Here's how the part is built. I have some questions about the finished solid (model axes, mm). A direction names the side the tool comes from. Give positions to 0.01 mm unless a question says otherwise; leave off trailing zeros. Order: outer loops, then holes, each group sorted by start corner. A loop starts at its lowest first (then second) coordinate and runs counter-clockwise, first axis right, second up.
from build123d import *

# Parameters (mm, degrees)
SKETCH1_R               = 8.2
BOSS_EXTRUDE1_DEPTH     = 72
SKETCH2_R               = 2.6
CUT_EXTRUDE1_DEPTH      = 6
CHAMFER1_SIZE           = 0.5
CHAMFER2_SIZE           = 1
SKETCH3_R               = 2.6
CUT_EXTRUDE2_DEPTH      = 33
CUT_EXTRUDE3_DEPTH      = 10
CUT_EXTRUDE4_DEPTH      = 2
CUT_EXTRUDE5_DEPTH      = 10
CUT_EXTRUDE5_DEPTH_BACK = 10
CUT_EXTRUDE6_DEPTH      = 9.232013
FILLET1_R               = 4
FILLET2_R               = 6
SKETCH9_R               = 2.6
CUT_EXTRUDE7_DEPTH      = 6
CHAMFER3_SIZE           = 0.5


with BuildPart() as part:
    # Sketch1 → Boss-Extrude1 (new body)
    with BuildSketch(Plane(origin=(0, 0, 0), x_dir=(1, 0, 0), z_dir=(0, 1, 0))):
        with BuildLine():
            Line((-16, 11), (16, 11))
            Line((16, 11), (16, -38))
            Line((16, -38), (10, -38))
            Line((10, -38), (10, -13.266499161))
            ThreePointArc((10, -13.266499161), (8.549193338, -10.697452646), (5.6, -10.613199329))
            ThreePointArc((5.6, -10.613199329), (-6.196773354, -10.276186063), (-12, 0))
            ThreePointArc((-12, 0), (-12.878679656, 2.121320344), (-15, 3))
            Line((-15, 3), (-16, 3))
            Line((-16, 3), (-16, 11))
        make_face()
        with Locations(Location((0, 0, 0), (0, 0, 270))):  # turned: the seam where the file's is
            Circle(SKETCH1_R, mode=Mode.SUBTRACT)
    extrude(amount=BOSS_EXTRUDE1_DEPTH)

    # Sketch2 → Cut-Extrude1 (cut)
    with BuildSketch(Plane.XY.offset(-11)):
        with Locations((-11, 67)):
            Circle(SKETCH2_R)
        with Locations((-11, 5)):
            Circle(SKETCH2_R)
        with Locations((11, 67)):
            Circle(SKETCH2_R)
        with Locations((11, 5)):
            Circle(SKETCH2_R)
    extrude(amount=CUT_EXTRUDE1_DEPTH, mode=Mode.SUBTRACT)

    # Chamfer1
    chamfer1_edges = [part.edges().sort_by_distance(p)[0] for p in [
        (-13.6, 67, -11),
        (-13.6, 5, -11),
        (8.4, 67, -11),
        (8.4, 5, -11),
    ]]
    chamfer(chamfer1_edges, length=CHAMFER1_SIZE)

    # Chamfer2
    chamfer2_edges = [part.edges().sort_by_distance(p)[0] for p in [
        (0, 0, -8.2),
        (0, 72, -8.2),
    ]]
    chamfer(chamfer2_edges, length=CHAMFER2_SIZE)

    # Sketch3 → Cut-Extrude2 (cut, through all)
    with BuildSketch(Plane(origin=(16, 0, 0), x_dir=(0, 0, -1), z_dir=(1, 0, 0))):
        with Locations((-29.75, 66)):
            Circle(SKETCH3_R)
        with Locations((-29.75, 58)):
            Circle(SKETCH3_R)
    extrude(amount=-CUT_EXTRUDE2_DEPTH, mode=Mode.SUBTRACT)

    # Sketch4 → Cut-Extrude3 (cut)
    with BuildSketch(Plane(origin=(0, 0, -11), x_dir=(-1, 0, 0), z_dir=(0, 0, -1))):
        with BuildLine():
            Line((-11, 72), (-16, 72))
            Line((-16, 72), (-16, 67))
            ThreePointArc((-16, 67), (-14.535533906, 70.535533906), (-11, 72))
        make_face()
    extrude(amount=-CUT_EXTRUDE3_DEPTH, mode=Mode.SUBTRACT)

    # Sketch5 → Cut-Extrude4 (cut)
    with BuildSketch(Plane(origin=(16, 0, 0), x_dir=(0, 0, -1), z_dir=(1, 0, 0))):
        Polygon((10.232013106, 51.021676305), (-14.652921151, 0), (-38, 0), (-38, 11.441867396), (-13.136632097, 62.419326121), (10.232013106, 62.419326121), align=None)
    extrude(amount=-CUT_EXTRUDE4_DEPTH, mode=Mode.SUBTRACT)

    # Sketch6 → Cut-Extrude5 (cut, two sides)
    with BuildSketch(Plane(origin=(14, 0, 0), x_dir=(0, 0, -1), z_dir=(1, 0, 0))) as cut_extrude5_sk:
        with BuildLine():
            Line((-38, 0), (-18, 0))
            Line((-18, 0), (-18, 25))
            ThreePointArc((-18, 25), (-19.464466094, 28.535533906), (-23, 30))
            Line((-23, 30), (-38, 30))
            Line((-38, 30), (-38, 0))
        make_face()
    extrude(amount=CUT_EXTRUDE5_DEPTH, mode=Mode.SUBTRACT)
    extrude(cut_extrude5_sk.sketch, amount=-CUT_EXTRUDE5_DEPTH_BACK, mode=Mode.SUBTRACT)

    # Sketch8 → Cut-Extrude6 (cut)
    with BuildSketch(Plane(origin=(0, 0, -1), x_dir=(-1, 0, 0), z_dir=(0, 0, -1))):
        Polygon((-16, 67), (-16, 62.419326121), (-14, 62.419326121), (-14, 63.535898385), align=None)
    extrude(amount=CUT_EXTRUDE6_DEPTH, mode=Mode.SUBTRACT)

    # Fillet1
    fillet1_edges = [part.edges().sort_by_distance(p)[0] for p in [
        (15, 62.419326121, -1),
    ]]
    fillet(fillet1_edges, radius=FILLET1_R)

    # Fillet2
    fillet2_edges = [part.edges().sort_by_distance(p)[0] for p in [
        (13, 72, 38),
    ]]
    fillet(fillet2_edges, radius=FILLET2_R)

    # Sketch9 → Cut-Extrude7 (cut)
    with BuildSketch(Plane(origin=(16, 0, 0), x_dir=(0, 0, -1), z_dir=(1, 0, 0))):
        with Locations((-18, 66)):
            Circle(SKETCH9_R)
        with Locations((5, 14)):
            Circle(SKETCH9_R)
    extrude(amount=-CUT_EXTRUDE7_DEPTH, mode=Mode.SUBTRACT)

    # Chamfer3
    chamfer3_edges = [part.edges().sort_by_distance(p)[0] for p in [
        (16, 66, 20.6),
        (16, 14, -2.4),
        (16, 66, 32.35),
        (16, 58, 32.35),
    ]]
    chamfer(chamfer3_edges, length=CHAMFER3_SIZE)


solid = part.part
Q1. I'm going to push flat-ended pins straight in: P1, Ø4, axis at x = 11, y = 67, coming from the -Z side; P2, Ø3, axis at y = 58, z = 29.75, coming from the +X side; P3, Ø2.5, axis at y = 14, z = -6, coming from the +X side; P4, Ø5, axis at x = 9, z = 28, coming from the -Y side. Where does each tip first touch, or does it pass through?
Filled sheet:
P1: stops at z = -5
P2: passes through
P3: stops at x = 10
P4: stops at y = 30
Q2. If we section it at D-D on y = 14: List the corners of the cut face in (x, z) for me.
Filled sheet:
outline: (-16, -11) - (16, -11) - (16, -8.1) - (15.5, -7.6) - (10, -7.6) - (10, -2.4) - (15.5, -2.4) - (16, -1.9) - (16, 7.82) - (14, 7.82) - (14, 18) - (10, 18) - (10, 13.27) arc R3 cw to (5.6, 10.61) arc R12 ccw to (-12, 0) arc R3 cw to (-15, -3) - (-16, -3) - close; hole circle Ø16.4 at (0, 0)
Q3. For faces 1 (the face through (12.79, 68.19, 16.6)), 2 (the face through (10, 14, -5)), 3 (the face through (-8.52, 5.78, -7.79)), which set-ups out of +Z, -Z, +X, -X, +Y, -Y let a thin tool reach every point of the face, with its end or its side?
Filled sheet:
face 1: +X, -X
face 2: +X
face 3: -Z
Q4. Thinking about a two-plate mould opening in Z: for faces 4 (the face through (-11, 5, -5)), 5 (the face through (14, 39, 9)), 6 (the face through (-12.86, 35.5, -2.1)), which applies, released by +Z, released by -Z, zero draft, split by the parting line, or undercut?
Filled sheet:
face 4: released by -Z
face 5: undercut
face 6: released by +Z
Q5. I need wall thicknesses on L1, parallel to Y at x = -11, z = -7.4; L2, parallel to Z at x = 2.5, y = 67; L3, parallel to Y at x = 11, z = -7.3. Which ranges of each line are inside material? Lowest first, please.
Filled sheet:
L1: y = 0 to 2.4, 7.6 to 64.4, 69.6 to 72
L2: z = -11 to -7.81, 7.81 to 11.74
L3: y = 0 to 2.4, 7.6 to 12.79, 15.21 to 64.4, 69.6 to 72
Q6. If we section it at B-B on z = 24.5: List the corners of the cut face in (x, y) for me, plus the area to 3 significant figures.
Filled sheet:
outline: (10, 30) - (14, 30) - (14, 39.12) - (16, 39.12) - (16, 72) - (10, 72) - close
area: 234 mm2
Q7. If we section it at C-C on z = 30: Give the number of separate pieces and of enclosed holes in the cut face, plus the area to 3 significant figures.
Filled sheet:
separate pieces: 3
enclosed holes: 0
area: 189 mm2
Q8. If we section it at A-A on y = 38: List the corners of the cut face in (x, z) for me, plus the area to 3 significant figures.
Filled sheet:
outline: (-16, -11) - (16, -11) - (16, -3.88) - (14, -3.88) - (14, 25.05) - (16, 25.05) - (16, 38) - (10, 38) - (10, 13.27) arc R3 cw to (5.6, 10.61) arc R12 ccw to (-12, 0) arc R3 cw to (-15, -3) - (-16, -3) - close; hole circle Ø16.4 at (0, 0)
area: 526 mm2
